from build123d import *

# Parameters (mm, degrees)
CROQUIS1_R              = 12.7
SALIENTE_EXTRUIR1_DEPTH = 20
CROQUIS2_R              = 12.7
CROQUIS3_R              = 12.25
SALIENTE_EXTRUIR2_DEPTH = 150
CROQUIS4_R              = 12.25


with BuildPart() as part:
    # Croquis1 → Saliente-Extruir1 (new body)
    with BuildSketch(Plane(origin=(0, 0, 0), x_dir=(1, 0, 0), z_dir=(0, 1, 0))):
        with Locations(Location((0, 0, 0), (0, 0, 270))):
            Circle(CROQUIS1_R)
    extrude(amount=SALIENTE_EXTRUIR1_DEPTH)

    # Barrer1: sweep along a curve in space
    with BuildLine() as barrer1_path:
        Line((0, 20, 0), (0, 340, 0))
        ThreePointArc((0, 340, 0), (0, 361.213203436, -8.786796564), (0, 370, -30))
        Line((0, 370, -30), (0, 370, -220))
        ThreePointArc((0, 370, -220), (-8.786796564, 370, -241.213203436), (-30, 370, -250))
        Line((-30, 370, -250), (-420, 370, -250))
        ThreePointArc((-420, 370, -250), (-441.213203436, 378.786796564, -250), (-450, 400, -250))
        Line((-450, 400, -250), (-450, 1325, -250))
    # Croquis2 → Barrer1 (sweep)
    with BuildSketch(Plane(origin=(0, 20, 0), x_dir=(1, 0, 0), z_dir=(0, 1, 0))):
        Circle(CROQUIS2_R)
    sweep(path=barrer1_path.line)

    # Croquis3 → Saliente-Extruir2 (add)
    with BuildSketch(Plane(origin=(0, 1325, 0), x_dir=(1, 0, 0), z_dir=(0, 1, 0))):
        with Locations(Location((-450, 250, 0), (0, 0, 270))):
            Circle(CROQUIS3_R)
    extrude(amount=SALIENTE_EXTRUIR2_DEPTH)

    # Barrer2: sweep along a curve in space
    with BuildLine() as barrer2_path:
        Line((-450, 1475, -250), (-450, 1525, -250))
        Line((-450, 1525, -250), (-510, 1525, -250))
    # Croquis4 → Barrer2 (sweep)
    with BuildSketch(Plane(origin=(0, 1475, 0), x_dir=(1, 0, 0), z_dir=(0, 1, 0))):
        with Locations((-450, 250)):
            Circle(CROQUIS4_R)
    sweep(path=barrer2_path.line, transition=Transition.RIGHT)


solid = part.part
Check sheet for the modelled part. Datum: model origin and axes. Units: mm. A direction names the side the tool comes from. Give positions to 0.01 mm unless a question says otherwise; leave off trailing zeros. Loops run counter-clockwise (first coordinate to the right, second up) from the corner with the lowest first, then second, coordinate; pieces in that order, holes last. Notation, with made-up numbers: M 32,89.5 L 49,89.5 A27 cw 49,118.5 Z; hole C -34.75,59 d8. An arc over 180 degrees is marked long. Answer as a JSON object with one key per item and string values. Group by question number.
Q1. Cross-section at B-B on z = -173. Record the cut outline in (x, y).
Q2. Access from +Z, -Z, +X, -X, +Y, -Y to the whole of each face (thin tool, end or side, straight path). Record for faces 1 (the flat face through (0, 0, 0)), 2 (the cylindrical face through (-227.73, 359.291, -256.827)).
Q3. Cross-section at A-A on x = -297.5. Record the cut outline in (y, z), then the cut area to 3 significant figures.
Q4. Material ranges on line 1 along Z through (x, y) = (-294, 380); line 2 along X through (y, z) = (1120, -242.5); line 3 along Z through (x, y) = (-457, 1466), recorded low to high. Write a range as [from, to].
Evaluation:
{
 "1": {"outline": "C 0,370 d25.4"},
 "2": {"face 1": "+Z, -Z, +X, -X, -Y", "face 2": "none"},
 "3": {"outline": "C 370,-250 d25.4", "area": "507 mm2"},
 "4": {"line 1": "z = [-257.83, -242.17]", "line 2": "x = [-460.25, -439.75]", "line 3": "z = [-260.05, -239.95]"}
}
